Source: CAD feature listing. Evaluate the final solid. Frame: model axes, mm. Give positions to 0.01 mm unless a question says otherwise; leave off trailing zeros. Order: outer loops, then holes, each group sorted by start corner. A loop starts at its lowest first (then second) coordinate and runs counter-clockwise, first axis right, second up. Notation, with made-up numbers: M 55,53 L 95,53 A13 cw 95,74 Z; hole C 49.25,58.25 d11. An arc over 180 degrees is marked long. Answer in a Markdown table with one row per item. Add a question column.
(1) Section query D-D, the plane x = -22. Return loops of the section in (y, z).
(2) Section query A-A, the plane y = 82.5. Return loops of the section in (x, z).
(3) Pin query (flat end, axial travel): P1, Ø1, axis at x = 13.5, z = -1, coming from the +Y side; P2, Ø1.5, axis at x = -9, z = 0, coming from the -Y side; P3, Ø2.5, axis at x = -48.79, y = 51.29, coming from the +Z side; P4, Ø1, axis at y = 8, z = -1, coming from the +X side. Return the tip coordinate at first contact, or that it passes through.
(4) Mould query, pull axis Y, two halves, no side actions, for faces 1 (the face through (90.61, 31.04, -0.04)), 2 (the face through (-76.767, 1.159, -0.035)), 3 (the face through (-1, 4, -2.5)), 4 (the face through (-67.4, -34.55, -0.03)). Classes: pulls with the +Y half, pulls with the -Y half, needs draft (parallel to the pull), parting line crosses it, or undercut.
(5) Section query B-B, the plane x = -80. Return loops of the section in (y, z), plus the area to 3 significant figures.
(6) Material intervals for line 1 along Y through (x, z) = (40, -0.5); line 2 along X through (y, z) = (-67, 0.35); line 3 along Y through (x, z) = (-1.5, 0.35), sorted ascending.
(7) Section query C-C, the plane z = -0.9. Count the separate pieces of the cut face and the enclosed holes in it, plus the area to 3 significant figures.
from build123d import *

# Parameters (mm, degrees)
SKETCH1_R             = 95
SKETCH1_R_2           = 1.5
SKETCH1_R_3           = 2
SKETCH1_R_4           = 3.5
BOSS_EXTRUDE1_DEPTH   = 5
BODY_MOVE_COPY1_ANGLE = 90


with BuildPart() as part:
    # Sketch1 → Boss-Extrude1 (new body)
    with BuildSketch(Plane(origin=(0, 0, 0), x_dir=(1, 0, 0), z_dir=(0, 1, 0))):
        Circle(SKETCH1_R)
        with Locations((48.790367902, 48.790367902)):
            Circle(SKETCH1_R_2, mode=Mode.SUBTRACT)
        with Locations((0, 40)):
            Circle(SKETCH1_R_3, mode=Mode.SUBTRACT)
        with Locations((40, 0)):
            Circle(SKETCH1_R_3, mode=Mode.SUBTRACT)
        with Locations((0, -40)):
            Circle(SKETCH1_R_3, mode=Mode.SUBTRACT)
        with Locations((-40, 0)):
            Circle(SKETCH1_R_3, mode=Mode.SUBTRACT)
        with Locations((48.790367902, -48.790367902)):
            Circle(SKETCH1_R_2, mode=Mode.SUBTRACT)
        with Locations((-48.790367902, -48.790367902)):
            Circle(SKETCH1_R_2, mode=Mode.SUBTRACT)
        with Locations((-48.790367902, 48.790367902)):
            Circle(SKETCH1_R_2, mode=Mode.SUBTRACT)
        with Locations((80, 0)):
            Circle(SKETCH1_R_4, mode=Mode.SUBTRACT)
        with Locations((69.282032303, -40)):
            Circle(SKETCH1_R_4, mode=Mode.SUBTRACT)
        with Locations((40, -69.282032303)):
            Circle(SKETCH1_R_4, mode=Mode.SUBTRACT)
        with Locations((0, -80)):
            Circle(SKETCH1_R_4, mode=Mode.SUBTRACT)
        with Locations((-40, -69.282032303)):
            Circle(SKETCH1_R_4, mode=Mode.SUBTRACT)
        with Locations((-69.282032303, -40)):
            Circle(SKETCH1_R_4, mode=Mode.SUBTRACT)
        with Locations((-80, 0)):
            Circle(SKETCH1_R_4, mode=Mode.SUBTRACT)
        with Locations((-69.282032303, 40)):
            Circle(SKETCH1_R_4, mode=Mode.SUBTRACT)
        with Locations((-40, 69.282032303)):
            Circle(SKETCH1_R_4, mode=Mode.SUBTRACT)
        with Locations((0, 80)):
            Circle(SKETCH1_R_4, mode=Mode.SUBTRACT)
        with Locations((40, 69.282032303)):
            Circle(SKETCH1_R_4, mode=Mode.SUBTRACT)
        with Locations((69.282032303, 40)):
            Circle(SKETCH1_R_4, mode=Mode.SUBTRACT)
    extrude(amount=BOSS_EXTRUDE1_DEPTH)


with BuildPart() as part_1:
    # Body-Move/Copy1: moved
    add(part.part.rotate(Axis((0, 2.5, 0), (1, 0, 0)), BODY_MOVE_COPY1_ANGLE))


solid = part_1.part
Values follow:
| question | item | result |
|---|---|---|
| 1 | outline | M -89.92,-2.5 L 94.92,-2.5 L 94.92,2.5 L -89.92,2.5 Z |
| 2 | outline | M -51.23,-2.5 L -3.5,-2.5 L -3.5,2.5 L -51.23,2.5 Z; M 3.5,-2.5 L 51.23,-2.5 L 51.23,2.5 L 3.5,2.5 Z |
| 3 | P1 | stops at y = 96.61 |
| 3 | P2 | stops at y = -92.14 |
| 3 | P3 | passes through |
| 3 | P4 | stops at x = 94.87 |
| 4 | face 1 | parting line crosses it |
| 4 | face 2 | undercut |
| 4 | face 3 | needs draft |
| 4 | face 4 | undercut |
| 5 | outline | M -48.73,-2.5 L -1,-2.5 L -1,2.5 L -48.73,2.5 Z; M 6,-2.5 L 53.73,-2.5 L 53.73,2.5 L 6,2.5 Z |
| 5 | area | 477 mm² |
| 6 | line 1 | y = -83.67 to -70.28, -63.28 to 0.5, 4.5 to 68.28, 75.28 to 88.67 |
| 6 | line 2 | x = -64.77 to -43.49, -36.51 to 36.51, 43.49 to 64.77 |
| 6 | line 3 | y = -92.49 to -80.66, -74.34 to -38.82, -36.18 to 41.18, 43.82 to 79.34, 85.66 to 97.49 |
| 7 | separate pieces | 1 |
| 7 | enclosed holes | 20 |
| 7 | area | 27,800 mm² |
